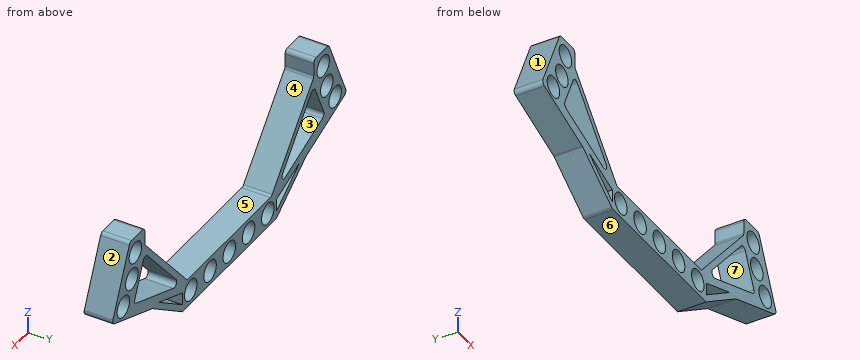
Autodesk Inventor part; units mm, degrees
ref_plane "YZ Plane" through (0, 0, 0) normal (1, 0, 0) x (0, 1, 0)
ref_plane "XZ Plane" through (0, 0, 0) normal (0, 1, 0) x (-1, 0, 0)
ref_plane "XY Plane" through (0, 0, 0) normal (0, 0, 1) x (1, 0, 0)
sketch "Sketch1" plane through (0, 0, 0) normal (0, 1, 0) x (-1, 0, 0)
  circle A0 centre (39, -6.055) radius 2.6
  circle A1 centre (40.5, -12.055) radius 2.6
  circle A2 centre (44, -17.055) radius 2.6
  line L0 (48.784, -18.8092) -> (41.3, -2)
  line L1 (0, 0) -> (60.8895, 0) construction
  line L2 (41.3, -2) -> (35.1, -2)
  circle A3 centre (16, -30.05) radius 2.6
  circle A4 centre (8, -30.05) radius 2.6
  arc A5 (0, -32.65) -> (0, -27.45) centre (0, -30.05) ccw
  line L3 (0, -33.55) -> (0, -32.65)
  line L4 (0, -27.45) -> (0, -26.55)
  line L5 (35.1, -2) -> (35.1, -6.5)
  line L6 (35.1, -8.7741) -> (39.6892, -19.0815)
  line L7 (0, -33.55) -> (19.5, -33.55)
  line L8 (19.5, -31.7318) -> (19.5, -28.6602)
  line L9 (19.5, -33.55) -> (31.902, -25.0543)
  line L10 (19.5, -31.7318) -> (29.2478, -25.0543)
  line L11 (17.5043, -26.55) -> (35.1, -6.5)
  line L12 (19.5, -26.55) -> (35.1, -8.7741)
  line L13 (19.5, -28.6602) -> (29.2478, -25.0543)
  line L14 (0, -26.55) -> (17.5043, -26.55)
  line L15 (39.6892, -19.0815) -> (19.5, -26.55)
  line L16 (48.784, -18.8092) -> (31.902, -25.0543)
  dimension "d0" = 5.2
  dimension "d1" = 1.5
  dimension "d3" = 3.5
  dimension "d5" = 6
  dimension "d6" = 5
  dimension "d12" = 39
  dimension "d14" = 114
  dimension "d15" = 18.4
  dimension "d16" = 6.055
  dimension "d17" = 6.2
  dimension "d19" = 30.05
  dimension "d21" = 8
  dimension "d22" = 5.2
  dimension "d26" = 3.9
  dimension "d29" = 19.5
  dimension "d31" = 18
  dimension "d35" = 1.5
  dimension "d37" = 1.5
  dimension "d40" = 3.5
  dimension "d41" = 3.5
  dimension "d44" = 4.5
  dimension "d45" = 0
  dimension "d46" = 8
  dimension "d48" = 2.9
  dimension "d49" = 2
  dimension "d51" = 0
extrude "Extrusion1" add sketch "Sketch1" along normal blind 7
mirror "Mirror1" about plane through (0, 0, -32.65) normal (1, 0, 0) of "Extrusion1"
fillet "Fillet1" radius 1 18 edges at (-35.1, 3.5, -8.7741) (-39.6892, 3.5, -19.0815) (-19.5, 3.5, -26.55) (19.5, 3.5, -26.55) (39.6892, 3.5, -19.0815) (35.1, 3.5, -8.7741) (48.784, 3.5, -18.8092) (41.3, 3.5, -2) (35.1, 3.5, -2) (35.1, 3.5, -6.5) (-17.5043, 3.5, -26.55) (-35.1, 3.5, -6.5) (-35.1, 3.5, -2) (-41.3, 3.5, -2) (-48.784, 3.5, -18.8092) (-31.902, 3.5, -25.0543) (-19.5, 3.5, -33.55) (31.902, 3.5, -25.0543)
equation "\"d37\" = d34"
equation "\"d41\" = d40"
equation "\"d46\" = d21"
equation "\"d34\" = d35"
properties part number "2020-04-02-10-10501-LED_Splitter_Transparent" material "ABS Plastic"
Model file for the job. Use its own axes, mm. Face numbers are marked on the shaded views. A direction names the side the tool comes from. Give positions to 0.01 mm unless a question says otherwise; leave off trailing zeros. Write each loop counter-clockwise with the first axis right and the second up, starting at its lowest first coordinate (ties: lowest second). Pieces come first, ordered by that corner, then holes. Notation, with made-up numbers: M 19,75.25 L 36,75.25 A35 cw 36,113.25 Z; hole C -7.75,20 d11. An arc over 180 degrees is marked long. Use a Markdown table: item, result.
1) Pin check, flat tips, straight feed: pin 1 (4 mm diameter, centred on x = -10, y = 2, fed in from +Z); pin 2 (1.5 mm diameter, centred on y = 4, z = -29.5, fed in from +X); pin 3 (3 mm diameter, centred on x = -39, z = -6.055, fed in from +Y); pin 4 (2.5 mm diameter, centred on y = 3, z = -5, fed in from +X). Stop position of each tip, or through.
Responses:
| item | result |
|---|---|
| pin 1 | stops at z = -26.55 |
| pin 2 | stops at x = 26.51 |
| pin 3 | passes through |
| pin 4 | stops at x = 43.19 |
2) Cut at B-B (x = 44). List the corners of the cut face in (y, z) (3 decimals).
Responses:
| item | result |
|---|---|
| outline | M 0,-20.579 L 7,-20.579 L 7,-19.655 L 0,-19.655 Z; M 0,-14.455 L 7,-14.455 L 7,-8.064 L 0,-8.064 Z |
3) Tool access for the marked faces 5, 6 and 7: list every direction of +Z, -Z, +X, -X, +Y, -Y with a clear straight run to the whole face (end or side of a thin tool).
Responses:
| item | result |
|---|---|
| face 5 | +Z, +Y, -Y |
| face 6 | -Z, +X, -X, +Y, -Y |
| face 7 | +Y, -Y |
4) Drill centre lines: line 1 (X direction, y = 4, z = -12.5); line 2 (Z direction, x = -37, y = 3.75); line 3 (X direction, y = 6.75, z = -32). Where is each one in solid material? Low to high. Write a range as from..to.
Responses:
| item | result |
|---|---|
| line 1 | x = -45.97..-43.06, -37.94..-36.76, -31.83..-29.83, 29.83..31.83, 36.76..37.94, 43.06..45.97 |
| line 2 | z = -23.17..-20.08, -13.04..-7.72, -4.39..-2 |
| line 3 | x = -21.76..-17.72, -14.28..-9.72, -6.28..-1.72, 1.72..6.28, 9.72..14.28, 17.72..21.76 |
5) Pull direction X, two halves, no side cores. Call the marked faces 1, 2, 3 and 4: +X half, -X half, draft (parallel to the pull), parting line (faces both ways), or undercut.
Responses:
| item | result |
|---|---|
| face 1 | -X half |
| face 2 | +X half |
| face 3 | undercut |
| face 4 | undercut |
6) Cut at A-A (x = 0). List the corners of the cut face in (y, z), and give its area (3 significant figures).
Responses:
| item | result |
|---|---|
| outline | M 0,-33.55 L 7,-33.55 L 7,-32.65 L 0,-32.65 Z; M 0,-27.45 L 7,-27.45 L 7,-26.55 L 0,-26.55 Z |
| area | 12.6 mm2 |
7) Cut at C-C (y = 2.75). Give the number of separate pieces and of enclosed holes in the cut face, and give its area (3 significant figures).
Responses:
| item | result |
|---|---|
| separate pieces | 1 |
| enclosed holes | 15 |
| area | 584 mm2 |
